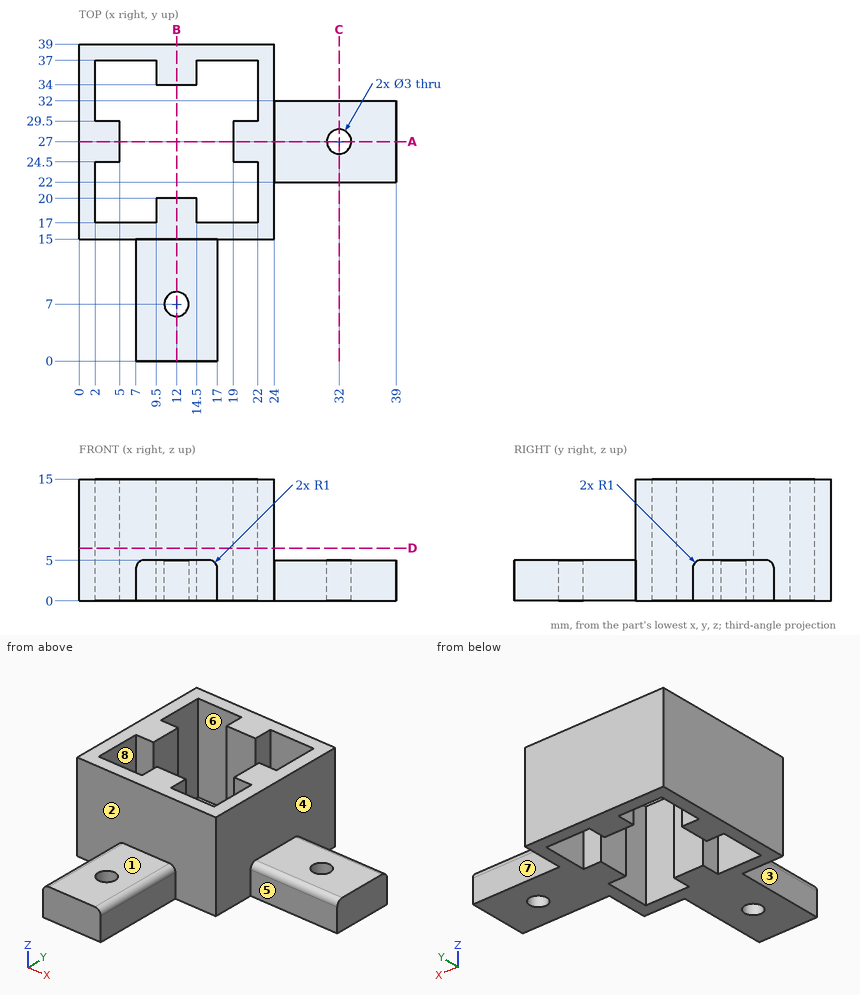
Geometry check sheet. Reference: drawing and pictorial views, mm from the part's lowest x, y, z. A direction names the side the tool comes from. Round coordinates to 2 decimals unless told otherwise and drop trailing zeros. Write each loop counter-clockwise with the first axis right and the second up, starting at its lowest first coordinate (ties: lowest second). Pieces come first, ordered by that corner, then holes.
1. Gauge pin test, flat ends, axial feed: P1, Ø2, axis at y = 8.5, z = 2, coming from the -X side; P2, Ø8, axis at x = 4.5, z = 11, coming from the -Y side; P3, Ø5, axis at y = 11.5, z = 12, coming from the +X side; P4, Ø1.2, axis at x = 28, z = 3, coming from the -Y side. Record the tip position at first contact, or that the pin passes through.
2. Draft check along Y on the marked faces 5, 6, 7 and 8. Enter one of: +Y half, -Y half, draft (parallel to the pull), parting line (faces both ways), or undercut.
3. Section check C-C on x = 32. Enter the section's corners in (y, z), plus the area to 3 significant figures.
4. Section check B-B on x = 12. Enter the section's corners in (y, z).
5. Access from +Z, -Z, +X, -X, +Y, -Y to the whole of each face (thin tool, end or side, straight path). Record for the marked faces 1, 2, 3 and 4.
6. Section check D-D on z = 6.5. Enter the section's corners in (x, y).
7. Section check A-A on y = 27. Enter the section's corners in (x, z), plus the area to 3 significant figures.
8. Scan lines: L1, parallel to X at y = 18, z = 12.5; L2, parallel to Y at x = 12, z = 3.6; L3, parallel to X at y = 27, z = 3.55. Record each from-to range of solid material in increasing order.
Answer:
1. P1: stops at x = 7
1. P2: stops at y = 15
1. P3: passes through
1. P4: stops at y = 22
2. face 5: -Y half
2. face 6: undercut
2. face 7: +Y half
2. face 8: undercut
3. outline: (22, 0) - (25.5, 0) - (25.5, 5) - (23, 5) arc R1 ccw to (22, 4) - close; (28.5, 0) - (32, 0) - (32, 4) arc R1 ccw to (31, 5) - (28.5, 5) - close
3. area: 34.6 mm2
4. outline: (0, 0) - (5.5, 0) - (5.5, 5) - (0, 5) - close; (8.5, 0) - (20, 0) - (20, 15) - (15, 15) - (15, 5) - (8.5, 5) - close; (34, 0) - (39, 0) - (39, 15) - (34, 15) - close
5. face 1: +Z, +X, -X, -Y
5. face 2: +Z, -Y
5. face 3: +Z, -Z, -X, -Y
5. face 4: +Z, +X
6. outline: (0, 15) - (24, 15) - (24, 39) - (0, 39) - close; hole (2, 17) - (9.5, 17) - (9.5, 20) - (14.5, 20) - (14.5, 17) - (22, 17) - (22, 24.5) - (19, 24.5) - (19, 29.5) - (22, 29.5) - (22, 37) - (14.5, 37) - (14.5, 34) - (9.5, 34) - (9.5, 37) - (2, 37) - (2, 29.5) - (5, 29.5) - (5, 24.5) - (2, 24.5) - close
7. outline: (0, 0) - (5, 0) - (5, 15) - (0, 15) - close; (19, 0) - (30.5, 0) - (30.5, 5) - (24, 5) - (24, 15) - (19, 15) - close; (33.5, 0) - (39, 0) - (39, 5) - (33.5, 5) - close
7. area: 210 mm2
8. L1: x = 0 to 2, 9.5 to 14.5, 22 to 24
8. L2: y = 0 to 5.5, 8.5 to 20, 34 to 39
8. L3: x = 0 to 5, 19 to 30.5, 33.5 to 39
